Geometry check sheet. Reference: the model listing, model coordinates, mm. A direction names the side the tool comes from. Round coordinates to 2 decimals unless told otherwise and drop trailing zeros. Write each loop counter-clockwise with the first axis right and the second up, starting at its lowest first coordinate (ties: lowest second). Pieces come first, ordered by that corner, then holes. Notation, with made-up numbers: (40.5, 19) - (99.5, 19) arc R22 ccw to (99.5, 25) - close; hole circle Ø8 at (-3, 19.25). An arc over 180 degrees is marked (long way). Return JSON: item names as keys, results as strings.
```python
from build123d import *

# Parameters (mm, degrees)
F1_DEPTH    = 5
F3_DEPTH    = 4
F4_W        = 15
F4_H        = 1
F4_W_2      = 20
F5_DEPTH    = 25
F6_T1_DEPTH = 6.2738947701
F6_T3_DEPTH = 7
F8_DEPTH    = 1
F9_T1_DEPTH = 1


# Not quite as in the source:
# - a fillet or chamfer that OpenCascade refuses, or shapes differently, is made with other operations: its cross-section is extruded or revolved along the edge and cut away or added


with BuildPart() as f1:
    # F0 (on Top) → F1 (new body)
    with BuildSketch(Plane.XY):
        with BuildLine():
            Line((38, 0), (0, 0))
            Line((0, 0), (0, -12))
            Line((0, -12), (38, -12))
            Line((38, -12), (38, -10.582575695))
            ThreePointArc((38, -10.582575695), (35, -6), (38, -1.417424305))
            Line((38, -1.417424305), (38, 0))
        make_face()
    extrude(amount=F1_DEPTH)

    # F2 (on face) → F3 (cut)
    with BuildSketch(Plane.XY.offset(5)):
        with BuildLine():
            ThreePointArc((38, -11.6568542495), (34, -6), (38, -0.3431457505))
            Line((38, -0.3431457505), (38, 0))
            Line((38, 0), (18, 0))
            Line((18, 0), (18, -1))
            Line((18, -1), (0, -1))
            Line((0, -1), (0, -11))
            Line((0, -11), (23, -11))
            Line((23, -11), (23, -12))
            Line((23, -12), (38, -12))
            Line((38, -12), (38, -11.6568542495))
        make_face()
    extrude(amount=-F3_DEPTH, mode=Mode.SUBTRACT)

    # F4 (on face) → F5 (cut)
    with BuildSketch(Plane(origin=(0, 0, 0), x_dir=(1, 0, 0), z_dir=(0, 0, -1))):
        with Locations((30.5, 11.5)):
            Rectangle(F4_W, F4_H)
        with Locations((28, 0.5)):
            Rectangle(F4_W_2, F4_H)
    extrude(amount=-F5_DEPTH, mode=Mode.SUBTRACT)

    # F6: fillet of radius 0.4 on 4 edges, made by hand

    # F6_s2 → F6_t1 (cut)
    with BuildSketch(Plane.XY.offset(-0.6369473851)):
        with BuildLine():
            ThreePointArc((37.7777777778, -10.4790320824), (37.9399346342, -10.6265361383), (38, -10.837354649))
            Line((38, -10.837354649), (38, -10.582575695))
            ThreePointArc((38, -10.582575695), (37.8882541717, -10.5321660998), (37.7777777778, -10.4790320824))
        make_face()
        with BuildLine():
            ThreePointArc((38, -1.162645351), (37.9399346342, -1.3734638617), (37.7777777778, -1.5209679176))
            ThreePointArc((37.7777777778, -1.5209679176), (37.8882541717, -1.4678339002), (38, -1.417424305))
            Line((38, -1.417424305), (38, -1.162645351))
        make_face()
    extrude(amount=F6_T1_DEPTH, mode=Mode.SUBTRACT)

    # F6_s4 → F6_t3 (cut)
    with BuildSketch(Plane.XY.offset(-1)):
        with BuildLine():
            ThreePointArc((38, -10.6), (37.8828427125, -10.8828427125), (37.6, -11))
            Line((37.6, -11), (38, -11))
            Line((38, -11), (38, -10.6))
        make_face()
        with BuildLine():
            ThreePointArc((38, -1.4), (37.8828427125, -1.1171572875), (37.6, -1))
            Line((37.6, -1), (38, -1))
            Line((38, -1), (38, -1.4))
        make_face()
    extrude(amount=F6_T3_DEPTH, mode=Mode.SUBTRACT)

    # F7 (on face) → F8 (cut)
    with BuildSketch(Plane.XY.offset(5)):
        with BuildLine():
            ThreePointArc((36.6833752096, -1), (34, -6), (36.6833752096, -11))
            Line((36.6833752096, -11), (37.6, -11))
            ThreePointArc((37.6, -11), (37.8372014652, -10.9220799045), (37.9819891264, -10.7186773245))
            ThreePointArc((37.9819891264, -10.7186773245), (37.9044539493, -10.5779171946), (37.7777777778, -10.4790320824))
            ThreePointArc((37.7777777778, -10.4790320824), (35, -6), (37.7777777778, -1.5209679176))
            ThreePointArc((37.7777777778, -1.5209679176), (37.9044539493, -1.4220828054), (37.9819891264, -1.2813226755))
            ThreePointArc((37.9819891264, -1.2813226755), (37.8372014652, -1.0779200955), (37.6, -1))
            Line((37.6, -1), (36.6833752096, -1))
        make_face()
    extrude(amount=-F8_DEPTH, mode=Mode.SUBTRACT)

    # F9: fillet of radius 5 on 2 edges, made by hand

    # F9_s2 → F9_t1 (join)
    with BuildSketch(Plane.XY):
        with BuildLine():
            ThreePointArc((18, 0), (19.4188611699, -0.7434164903), (21, -1))
            Line((21, -1), (18, -1))
            Line((18, -1), (18, 0))
        make_face()
        with BuildLine():
            ThreePointArc((26, -11), (24.4188611699, -11.2565835097), (23, -12))
            Line((23, -12), (23, -11))
            Line((23, -11), (26, -11))
        make_face()
    extrude(amount=F9_T1_DEPTH)


solid = f1.part
```
(1) Section check D-D, the plane z = 0.45. Enter the section's corners in (x, y).
Response values:
{"outline": "(0, -12) - (23, -12) arc R5 cw to (26, -11) - (37.6, -11) arc R0.4 ccw to (37.98, -10.72) arc R0.4 ccw to (37.78, -10.48) arc R5 cw to (37.78, -1.52) arc R0.4 ccw to (37.98, -1.28) arc R0.4 ccw to (37.6, -1) - (21, -1) arc R5 cw to (18, 0) - (0, 0) - close"}
(2) Release check for a two-part mould opening along Y. For faces 1 (the face through (9, -1, 3)), 2 (the face through (0, -5.9, 0.8)), 3 (the face through (11, -12, 2)), 4 (the face through (9, 0, 2)) record: pulls with the +Y half, pulls with the -Y half, needs draft (parallel to the pull), parting line crosses it, or undercut.
Response values:
{"face 1": "undercut", "face 2": "needs draft", "face 3": "pulls with the -Y half", "face 4": "pulls with the +Y half"}
(3) Section check A-A, the plane z = 2.95. Enter the section's corners in (x, y).
Response values:
{"outline": "(0, -12) - (23, -12) - (23, -11) - (0, -11) - close; (0, -1) - (18, -1) - (18, 0) - (0, 0) - close; (36.68, -11) - (37.6, -11) arc R0.4 ccw to (37.98, -10.72) arc R0.4 ccw to (37.78, -10.48) arc R5 cw to (37.78, -1.52) arc R0.4 ccw to (37.98, -1.28) arc R0.4 ccw to (37.6, -1) - (36.68, -1) arc R6 ccw to start"}
(4) Gauge pin test, flat ends, axial feed: pin 1 (2 mm diameter, centred on x = 29.5, y = -8.5, fed in from +Z); pin 2 (3 mm diameter, centred on x = 32.5, z = 2, fed in from +Y); pin 3 (0.5 mm diameter, centred on y = -0.5, z = 2, fed in from +X). Record the tip position at first contact, or that the pin passes through.
Response values:
{"pin 1": "stops at z = 1", "pin 2": "stops at y = -1", "pin 3": "stops at x = 18"}
(5) Material ranges on line 1 along Y through (x, z) = (15.5, 2.1); line 2 along Z through (x, y) = (30, -10.5); line 3 along Y through (x, z) = (19.5, 1.15), recorded low to high. Write a range as [from, to].
Response values:
{"line 1": "y = [-12, -11], [-1, 0]", "line 2": "z = [0, 1]", "line 3": "y = [-12, -11]"}
(6) Section check B-B, the plane z = 4.65. Enter the section's corners in (x, y), plus the area to 3 significant figures.
Response values:
{"outline": "(0, -12) - (23, -12) - (23, -11) - (0, -11) - close; (0, -1) - (18, -1) - (18, 0) - (0, 0) - close", "area": "41.0 mm^2"}
(7) Section check C-C, the plane x = 14. Enter the section's corners in (y, z), plus the area to 3 significant figures.
Response values:
{"outline": "(-12, 0) - (0, 0) - (0, 5) - (-1, 5) - (-1, 1) - (-11, 1) - (-11, 5) - (-12, 5) - close", "area": "20.0 mm^2"}
(8) Access from +Z, -Z, +X, -X, +Y, -Y to the whole of each face (thin tool, end or side, straight path). Record for faces 5 (the face through (32.6, -11, 0.7)), 6 (the face through (18, -0.5, 3)), 7 (the face through (29.9, -1, 0.7)).
Response values:
{"face 5": "+Z, -Z, +X, -Y", "face 6": "+Z, +X, +Y", "face 7": "+Z, -Z, +X, +Y"}
